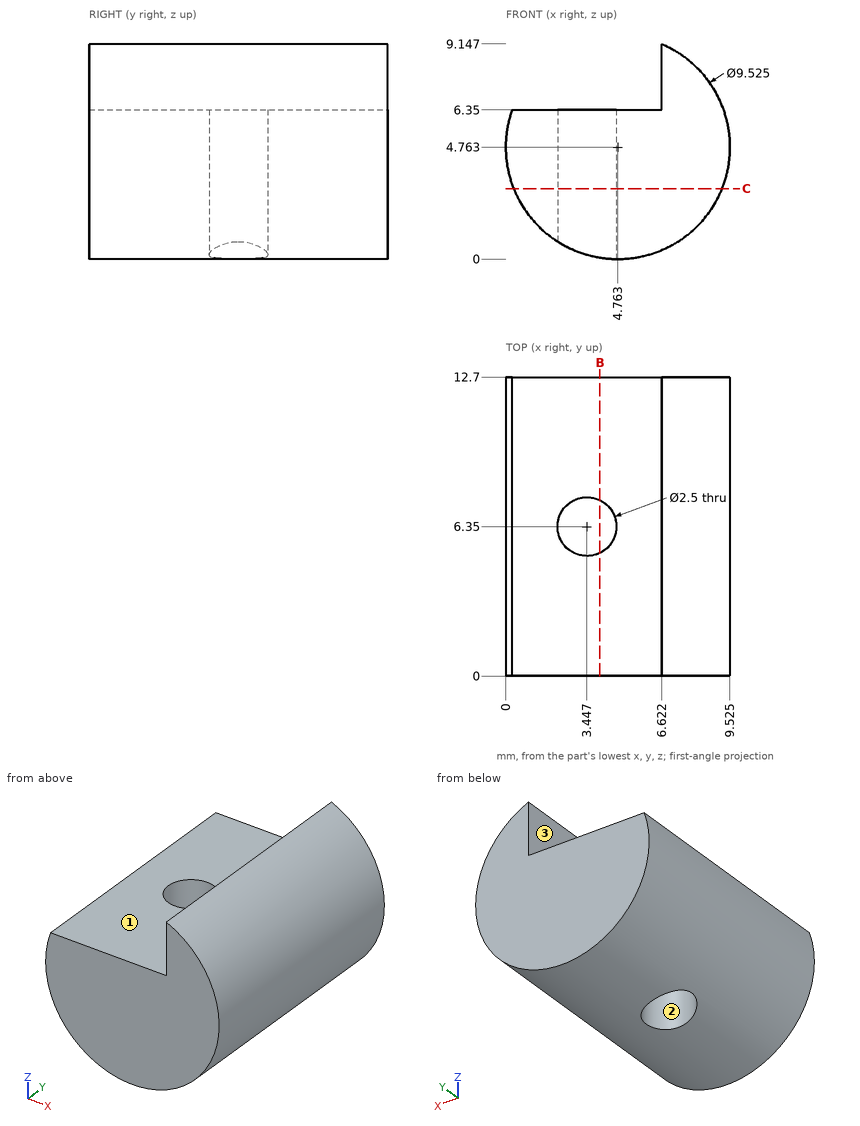
Geometry: see drawing. Coordinates: mm, zero at the bounding-box minimum. Coordinates: 2 decimals unless noted, no trailing zeros. Loops run counter-clockwise (first coordinate to the right, second up) from the corner with the lowest first, then second, coordinate; pieces in that order, holes last.
(1) First-contact query: pin 1 Ø1.5 at (x, y) = (3.45, 6.35) entering from -Z; pin 2 Ø1.5 at (y, z) = (7, 5.5) entering from -X; pin 3 Ø3 at (x, y) = (4, 4.5) entering from +Z; pin 4 Ø0.8 at (y, z) = (5, 7.5) entering from -X. Flat tips, straight axial feed; report the tip coordinate or a pass-through.
(2) Section C-C on z = 3. Return the cut outline in (x, y).
(3) Section B-B on x = 4. Return the cut outline in (y, z).
(4) Material intervals for probe 1 along Y at (x, z) = (3.5, 6.25); probe 2 along Z at (x, y) = (4.75, 9); probe 3 along X at (y, z) = (7, 1) (1 decimal), sorted ascending.
(5) Pull-direction query (X, two-part tool) for the marked faces 1, 2 and 3; classes: released by +X, released by -X, zero draft, split by the parting line, or undercut.
Data:
1. pin 1: passes through
1. pin 2: stops at x = 0
1. pin 3: stops at z = 6.35
1. pin 4: stops at x = 6.62
2. outline: (0.34, 0) - (9.19, 0) - (9.19, 12.7) - (0.34, 12.7) - close; hole circle Ø2.5 at (3.45, 6.35)
3. outline: (0, 0.06) - (5.23, 0.06) - (5.23, 6.35) - (0, 6.35) - close; (7.47, 0.06) - (12.7, 0.06) - (12.7, 6.35) - (7.47, 6.35) - close
4. probe 1: y = 0 to 5.1, 7.6 to 12.7
4. probe 2: z = 0 to 6.35
4. probe 3: x = 1.8 to 2.4, 4.5 to 7.7
5. face 1: zero draft
5. face 2: undercut
5. face 3: released by -X
